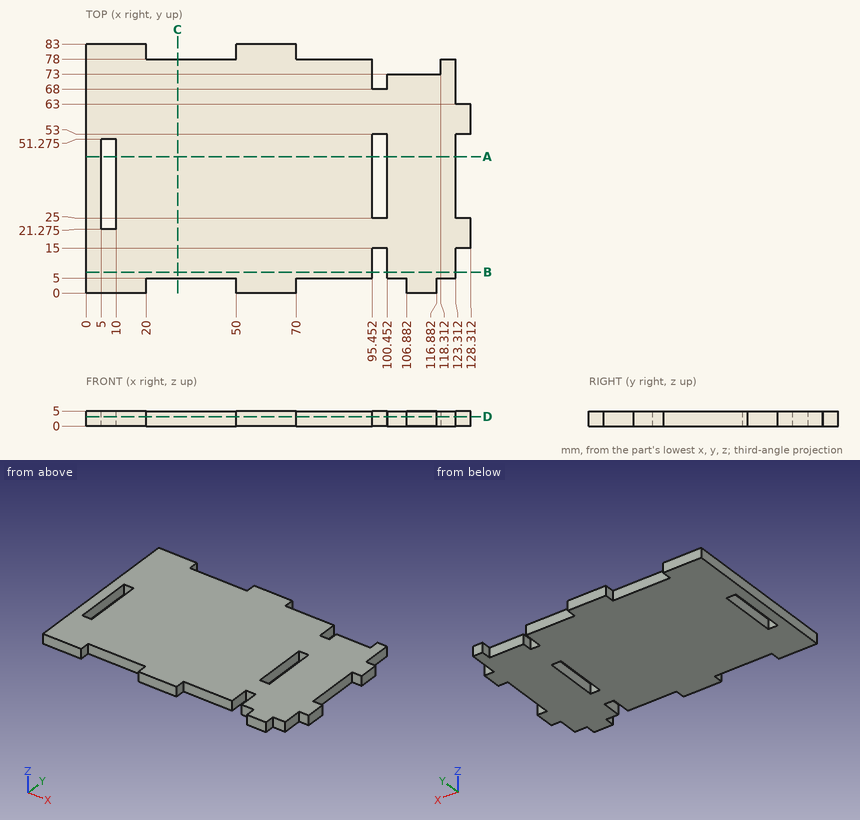
The drawing under review shows one solid part. Ordinate dimensions are in mm from its lowest x, y, z. Give positions to 0.01 mm unless a question says otherwise; leave off trailing zeros. Write each loop counter-clockwise with the first axis right and the second up, starting at its lowest first coordinate (ties: lowest second). Pieces come first, ordered by that corner, then holes. Notation, with made-up numbers: (9, 83.5) - (27, 83.5) arc R19 cw to (27, 119.5) - close; hole circle Ø11 at (71.25, -9.5). An arc over 180 degrees is marked (long way). Answer in a Markdown table with one row per item. Add a question column.
1. We need section B-B on y = 7. Write out the cut boundary in (x, z).
2. We need section A-A on y = 45.5. Write out the cut boundary in (x, z).
3. Wall thickness on line 1 along X through (y, z) = (32.5, 1.95); line 2 along X through (y, z) = (11, 2.8); line 3 along X through (y, z) = (23, 2.75): over which ranges is each line inside the solid? List them lowest first. Write a range as [from, to].
4. Insertion check: P1, Ø2.5, axis at x = 98.5, z = 2.5, coming from the +Y side; P2, Ø2.5, axis at y = 44.5, z = 2.5, coming from the +X side; P3, Ø1.5, axis at x = 34.5, z = 3, coming from the -Y side. Each pin has a flat end and moves straight along its axis. Give the tip position at first contact, or say it passes through.
5. We need section C-C on x = 30.5. Write out the cut boundary in (y, z).
6. We need section D-D on z = 3.1. State how many separate pieces and enclosed holes the cut face has, then the cut area to 3 significant figures.
Ans:
| question | item | result |
|---|---|---|
| 1 | outline | (0, 0) - (95.45, 0) - (95.45, 5) - (0, 5) - close; (100.45, 0) - (123.31, 0) - (123.31, 5) - (100.45, 5) - close |
| 2 | outline | (0, 0) - (5, 0) - (5, 5) - (0, 5) - close; (10, 0) - (95.45, 0) - (95.45, 5) - (10, 5) - close; (100.45, 0) - (123.31, 0) - (123.31, 5) - (100.45, 5) - close |
| 3 | line 1 | x = [0, 5], [10, 95.45], [100.45, 123.31] |
| 3 | line 2 | x = [0, 95.45], [100.45, 123.31] |
| 3 | line 3 | x = [0, 5], [10, 128.31] |
| 4 | P1 | stops at y = 68 |
| 4 | P2 | stops at x = 123.31 |
| 4 | P3 | stops at y = 5 |
| 5 | outline | (5, 0) - (78, 0) - (78, 5) - (5, 5) - close |
| 6 | separate pieces | 1 |
| 6 | enclosed holes | 2 |
| 6 | area | 9,070 mm^2 |
